```python
from build123d import *

# Parameters (mm, degrees)
EXTRUDE_1_DEPTH = 2
FILLET_1_R      = 2
SKETCH_5_W      = 25.102776666
SKETCH_5_H      = 0.92
EXTRUDE_2_DEPTH = 2


with BuildPart() as part:
    # 草图1 → 凸台-拉伸1 (new body)
    with BuildSketch(Plane.XY):
        Polygon((-8.301811847, -11.701358885), (-3.301811847, -11.701358885), (-3.301811847, -41.701358885), (13.698188153, -41.701358885), (13.698188153, -9.223166137), (34.95900929, -9.223166137), (34.95900929, 9.348641115), (13.698188153, 9.348641115), (7.098188153, 17.348641115), (-3.301811847, 17.348641115), (-3.301811847, 9.348641115), (0.698188153, 9.348641115), (0.698188153, 10.798641115), (3.898188153, 10.798641115), (3.898188153, 9.348641115), (7.098188153, 9.348641115), (7.098188153, 5.248641115), (3.898188153, 5.248641115), (3.898188153, 3.798641115), (0.698188153, 3.798641115), (0.698188153, 5.248641115), (-3.301811847, 5.248641115), (-3.301811847, -3.701358885), (-8.301811847, -3.701358885), align=None)
        with BuildLine():
            Line((0.698188153, -25.451358885), (8.698188153, -25.451358885))
            ThreePointArc((8.698188153, -25.451358885), (9.948188153, -26.701358885), (8.698188153, -27.951358885))
            Line((8.698188153, -27.951358885), (0.698188153, -27.951358885))
            ThreePointArc((0.698188153, -27.951358885), (-0.551811847, -26.701358885), (0.698188153, -25.451358885))
        make_face(mode=Mode.SUBTRACT)
        with BuildLine():
            Line((8.698188153, -37.451358885), (0.698188153, -37.451358885))
            ThreePointArc((0.698188153, -37.451358885), (-0.551811847, -36.201358885), (0.698188153, -34.951358885))
            Line((0.698188153, -34.951358885), (8.698188153, -34.951358885))
            ThreePointArc((8.698188153, -34.951358885), (9.948188153, -36.201358885), (8.698188153, -37.451358885))
        make_face(mode=Mode.SUBTRACT)
        with BuildLine():
            Line((32.20900929, 3.348641115), (32.20900929, -4.651358885))
            ThreePointArc((32.20900929, -4.651358885), (30.95900929, -5.901358885), (29.70900929, -4.651358885))
            Line((29.70900929, -4.651358885), (29.70900929, 3.348641115))
            ThreePointArc((29.70900929, 3.348641115), (30.95900929, 4.598641115), (32.20900929, 3.348641115))
        make_face(mode=Mode.SUBTRACT)
        with BuildLine():
            Line((22.70900929, 3.348641115), (22.70900929, -4.651358885))
            ThreePointArc((22.70900929, -4.651358885), (21.45900929, -5.901358885), (20.20900929, -4.651358885))
            Line((20.20900929, -4.651358885), (20.20900929, 3.348641115))
            ThreePointArc((20.20900929, 3.348641115), (21.45900929, 4.598641115), (22.70900929, 3.348641115))
        make_face(mode=Mode.SUBTRACT)
    extrude(amount=EXTRUDE_1_DEPTH)

    # 圆角1
    fillet_1_edges = [part.edges().sort_by_distance(p)[0] for p in [
        (-8.301811847, -3.701358885, 1),
        (-8.301811847, -11.701358885, 1),
    ]]
    fillet(fillet_1_edges, radius=FILLET_1_R)

    # 草图5 → 凸台-拉伸2 (add)
    with BuildSketch(Plane.XY.offset(2)):
        with Locations((22.407620957, 9.808641115)):
            Rectangle(SKETCH_5_W, SKETCH_5_H)
    extrude(amount=-EXTRUDE_2_DEPTH)


solid = part.part
```
CAD build for the part. Positions are in the model's coordinates, mm. A direction names the side the tool comes from. Give positions to 0.01 mm unless a question says otherwise; leave off trailing zeros. Write each loop counter-clockwise with the first axis right and the second up, starting at its lowest first coordinate (ties: lowest second). Pieces come first, ordered by that corner, then holes. Notation, with made-up numbers: (-12, 37) -> (34, 37) arc R11 cw to (34, 58) -> close; hole circle Ø5 at (86.5, 81.5). An arc over 180 degrees is marked (long way). Write each question's results on one line, items separated by ' | '.
1. Cut at D-D, the plane x = 17.5. Write the cut outline in (y, z).
Geometry check:
outline: (-9.22, 0) -> (10.27, 0) -> (10.27, 2) -> (-9.22, 2) -> close
2. Drop flat-ended pins along their axis: P1, Ø0.6, axis at y = -27.5, z = 1, coming from the +X side; P2, Ø0.7, axis at y = 10.5, z = 1, coming from the +X side; P3, Ø1, axis at x = -5, z = 1.5, coming from the -Y side; P4, Ø0.6, axis at y = 13, z = 0.5, coming from the -X side. Give the stop position or say it passes through.
Geometry check:
P1: x = 13.7 | P2: x = 34.96 | P3: y = -11.7 | P4: x = -3.3
3. Two-plate mould, pull along Y, no slides. Class faces 6 (the cylindrical face through (-7.7, -11.13, 1.01)), 7 (the flat face through (6, 5.249, 1)), 8 (the flat face through (24, 10.269, 1)): pulls with the +Y half, pulls with the -Y half, needs draft (parallel to the pull), parting line crosses it, or undercut.
Geometry check:
face 6: pulls with the -Y half | face 7: undercut | face 8: pulls with the +Y half
4. Wall check: probe 1 along Y at (x, z) = (6, 0.85); probe 2 along Y at (x, z) = (1, 1.65); probe 3 along X at (y, z) = (-3, 0.5). Give the ranges that are in metal, low to high. Write a range as [from, to].
Geometry check:
probe 1: [-41.7, -37.45], [-34.95, -27.95], [-25.45, 5.25], [9.35, 17.35] | probe 2: [-41.7, -37.45], [-34.95, -27.95], [-25.45, 3.8], [10.8, 17.35] | probe 3: [-3.3, 20.21], [22.71, 29.71], [32.21, 34.96]
5. Cut at C-C, the plane z = 0.4. Give the number of separate pieces and of enclosed holes in the cut face, then the cut area to 3 significant figures.
Geometry check:
separate pieces: 1 | enclosed holes: 4 | area: 1,280 mm²
6. Which spindle directions (+Z, -Z, +X, -X, +Y, -Y) get a long thin tool onto all of the face, cutting with end or side? Do faces 1 (the flat face through (34.959, 0, 1)), 2 (the flat face through (-3.302, 13, 1)), 3 (the flat face through (-1, 5.249, 1)), 4 (the flat face through (32.209, -1, 1)), 5 (the flat face through (-3.302, -26, 1)). Say none if no direction does.
Geometry check:
face 1: +Z, -Z, +X, +Y, -Y | face 2: +Z, -Z, -X, +Y | face 3: +Z, -Z, -X | face 4: +Z, -Z | face 5: +Z, -Z, -X, -Y
7. Cut at A-A, the plane y = 2.5. Write the cut outline in (x, z), then the cut area to 3 significant figures.
Geometry check:
outline: (-3.3, 0) -> (20.21, 0) -> (20.21, 2) -> (-3.3, 2) -> close; (22.71, 0) -> (29.71, 0) -> (29.71, 2) -> (22.71, 2) -> close; (32.21, 0) -> (34.96, 0) -> (34.96, 2) -> (32.21, 2) -> close | area: 66.5 mm²
8. Cut at B-B, the plane x = 31. Write the cut outline in (y, z).
Geometry check:
outline: (-9.22, 0) -> (-5.9, 0) -> (-5.9, 2) -> (-9.22, 2) -> close; (4.6, 0) -> (10.27, 0) -> (10.27, 2) -> (4.6, 2) -> close
